The model under review builds one solid part; all positions refer to its coordinate system, in mm. A direction names the side the tool comes from. Round coordinates to 2 decimals unless told otherwise and drop trailing zeros. Order: outer loops, then holes, each group sorted by start corner. A loop starts at its lowest first (then second) coordinate and runs counter-clockwise, first axis right, second up.
Autodesk Inventor part; units mm, degrees
ref_plane "YZ Plane" through (0, 0, 0) normal (1, 0, 0) x (0, 1, 0)
ref_plane "XZ Plane" through (0, 0, 0) normal (0, 1, 0) x (-1, 0, 0)
ref_plane "XY Plane" through (0, 0, 0) normal (0, 0, 1) x (1, 0, 0)
sketch "Skizze1" plane through (0, 0, 0) normal (0, 0, 1) x (1, 0, 0)
  line L0 (2.7, 9.6) -> (2.7, 4)
  arc A0 (2.7, 9.6) -> (2.2, 10.1) centre (2.2, 9.6) ccw
  line L1 (-0.6, 10.1) -> (2.2, 10.1)
  line L2 (-2.3, 10.1) -> (-0.6, 10.1)
  line L3 (-2.3, 10.1) -> (-2.3, 9.1)
  line L4 (-2.3, 9.1) -> (-2.3, 0)
  line L5 (-2.3, 0) -> (-2.3, -1)
  line L6 (-0.6, -1) -> (-2.3, -1)
  line L7 (-0.6, -0.995) -> (0, -0.995)
  line L8 (5.3, -1) -> (-0.6, -1)
  arc A1 (5.3, -1) -> (6.3, 0) centre (5.3, 0) ccw
  line L9 (6.3, 3) -> (6.3, 0)
  arc A2 (6.3, 3) -> (5.3, 4) centre (5.3, 3) ccw
  line L10 (2.7, 4) -> (5.3, 4)
  point P0 (0, 0)
extrude "Extrusion1" add sketch "Skizze1" along normal blind 10.2
sketch "Skizze2" plane through (-2.3, 10.1, 0) normal (0, 1, 0) x (1, 0, 0)
  line L0 (0, -10.2) -> (4.5, -10.2)
  line L1 (0, 0) -> (0, -10.2)
  line L2 (2.3, 0) -> (2.3, -0.9)
  line L3 (2.3, -0.9) -> (1.7, -0.9)
  line L4 (1.7, -0.9) -> (1.7, -1.5)
  line L5 (1.7, -1.5) -> (8.6, -1.5)
  line L6 (8.6, 0) -> (8.6, -10.2)
  line L7 (2.3, -10.2) -> (2.3, -9.3)
  line L8 (2.3, -9.3) -> (1.7, -9.3)
  line L9 (1.7, -9.3) -> (1.7, -8.7)
  line L10 (1.7, -8.7) -> (8.6, -8.7)
  line L11 (8.6, -1.5) -> (8.6, 0)
  line L12 (2.3, 0) -> (8.6, 0)
  line L13 (2.3, -10.2) -> (8.6, -10.2)
  line L14 (8.6, -8.7) -> (8.6, -10.2)
  dimension "d2" = 0.9
  dimension "d3" = 0.6
  dimension "d4" = 0.9
  dimension "d5" = 0.6
  dimension "d6" = 2.3
  dimension "d7" = 2.3
  dimension "d8" = 1.7
  dimension "d9" = 0.6
  dimension "d10" = 1.7
extrude "Extrusion2" cut sketch "Skizze2" against normal blind 12
sketch "Skizze3" plane through (2.7, 4, 8.7) normal (1, 0, 0) x (0, 0, -1)
  line L0 (0, 5.6) -> (0, 0)
  line L1 (7.2, 0) -> (0, 0)
  line L2 (7.2, 0) -> (7.2, 5.6)
  line L3 (7.2, 5.6) -> (0, 5.6)
  line L4 (7.2, 6.1) -> (0, 6.1)
  line L5 (-1.5, -5) -> (-1.5, 6.1)
  point P0 (8.7, -4)
  point P1 (3.55, 2.55)
  dimension "d13" = 3.55
  dimension "d14" = 5.05
sketch "Skizze4" plane through (-2.3, -1, 0) normal (-1, 0, 0) x (0, 0, 1)
  line L0 (10.2, 0) -> (10.2, 11.1)
  line L1 (0, 11.1) -> (10.2, 11.1)
  line L2 (0, 0) -> (0, 11.1)
  line L3 (10.2, 11.1) -> (10.2, 0)
  line L4 (10.2, 0) -> (0, 0)
  line L5 (0, 0) -> (0, 11.1)
  line L6 (0, 11.1) -> (10.2, 11.1)
  line L7 (10.2, 11.1) -> (10.2, 0)
  line L8 (10.2, 0) -> (0, 0)
  line L9 (0, 0) -> (0, 11.1)
  line L10 (0, 11.1) -> (10.2, 11.1)
  line L11 (10.2, 0) -> (10.2, 11.1)
  line L12 (0, 11.1) -> (10.2, 11.1)
  line L13 (0, 0) -> (0, 11.1)
  line L14 (0, 0) -> (10.2, 0)
  line L15 (8.7, 10.6) -> (8.7, 5)
  line L16 (1.5, 5) -> (8.7, 5)
  line L17 (1.5, 5) -> (1.5, 10.6)
  line L18 (1.5, 10.6) -> (8.7, 10.6)
  point P0 (0, 1)
  point P1 (5.1, 7.55)
  dimension "d15" = 3.55
  dimension "d16" = 5.1
  dimension "d17" = 5.1
hole "Hole1" at (-2.3, 6.55, 5.1) direction (1, 0, 0) diameter 2.013 end through all countersink diameter 4 countersink angle 90
sketch "Skizze5" plane through (2.2, 10.1, 1.5) normal (0, 0, -1) x (-1, 0, 0)
  line L0 (-4.1, -10.1) -> (-4.1, -7.1)
  line L1 (2.8, -11.1) -> (-3.1, -11.1)
  line L2 (-3.1, -6.1) -> (-0.5, -6.1)
  line L3 (2.2, 0) -> (2.2, -11.1)
  point P0 (2.2, -10.1)
  point P1 (-1.6, -8.6)
  dimension "d25" = 2.5
  dimension "d26" = 2.5
  dimension "d27" = 2.5
  dimension "d28" = 3.8
sketch "Skizze6" plane through (-0.6, 10.1, 8.7) normal (0, 0, 1) x (1, 0, 0)
  line L0 (6.9, -7.1) -> (6.9, -10.1)
  line L1 (3.3, -6.1) -> (5.9, -6.1)
  line L2 (0.6, -11.1) -> (0.6, 0)
  point P0 (0.6, -10.1)
  point P1 (4.4, -8.6)
  dimension "d29" = 2.5
  dimension "d30" = 2.5
  dimension "d31" = 3.8
hole "Hole2" at (3.8, 1.5, 8.7) direction (0, 0, -1) diameter 2.013 depth 6 tip angle 118 countersink diameter 4 countersink angle 90
hole "Hole3" at (3.8, 1.5, 1.5) direction (0, 0, 1) diameter 2.013 depth 6 tip angle 118 countersink diameter 4 countersink angle 90
sketch "Skizze7" plane through (-2.3, 10.1, 10.2) normal (0, 1, 0) x (1, 0, 0)
  line L0 (0, 10.2) -> (2.3, 10.2)
  line L1 (0, 10.2) -> (0, 0)
  line L2 (0, 0) -> (2.3, 0)
  line L3 (0, 7.65) -> (0.2, 7.65)
  line L4 (0.2, 7.65) -> (0.2, 2.55)
  line L5 (0.2, 2.55) -> (0, 2.55)
  line L6 (0, 7.65) -> (0, 2.55)
  dimension "d46" = 2.55
  dimension "d47" = 2.55
  dimension "d48" = 0.2
extrude "Extrusion3" cut sketch "Skizze7" against normal blind 12
fillet "Rundung1" radius 0.5 1 edges at (-1.15, 10.1, 10.2)
fillet "Rundung2" radius 0.5 3 edges at (-1.15, 10.1, 0) (-1.15, -1, 0) (-1.15, -1, 10.2)
properties part number "4. Leiterplattenhalter_Links"
(1) We need section D-D (z = 8). Give the boundary of the cut face in (x, y), and give its area (3 significant figures).
(2) We need section A-A (y = 1.5). Give the boundary of the cut face in (x, z), and give its area (3 significant figures).
(3) To check wall thickness, follow L1, parallel to Y at x = 3.8, z = 7.6; L2, parallel to Z at x = -0.5, y = 7; L3, parallel to Y at x = -0.3, z = 5.1. State the ranges of each line that lie inside material, in increasing order.
(4) Clearance check with flat-ended pins moving along their axes: P1, Ø3.5, axis at x = 3, y = 2.5, coming from the -Z side; P2, Ø0.7, axis at y = 3.5, z = 1, coming from the +X side; P3, Ø1.5, axis at y = 2, z = 4.5, coming from the -X side. State where each tip first meets the part, or that it passes through.
(5) We need section C-C (x = 1.25). Give the boundary of the cut face in (y, z), and give its area (3 significant figures).
(6) We need section B-B (z = 5.1). Give the boundary of the cut face in (x, y), and give its area (3 significant figures).
(7) The part is to be moulded in two halves that separate along Z. For faces 1 (the flat face through (0, 10.1, 5)), 2 (the cylindrical face through (1, 7, 6)), 3 (the flat face through (-1, 5, 10.2)), 4 (the flat face through (1, 5, 1.5)), say which applies: pulls with the +Z half, pulls with the -Z half, needs draft (parallel to the pull), parting line crosses it, or undercut.
(8) Tool access review of faces 5 (the flat face through (0, 5, 10)), 6 (the flat face through (-2.1, 4.6, 5.1)), 7 (the flat face through (6.3, 2, 5)), 8 (the flat face through (4, 4, 5)), 9 (the flat face through (0, 4.6, 0.4)): name each direction out of +Z, -Z, +X, -X, +Y, -Y from which nothing blocks a thin tool from reaching the whole face with its end or side.
Verdict:
1. outline: (-2.3, -1) - (5.3, -1) arc R1 ccw to (6.3, 0) - (6.3, 3) arc R1 ccw to (5.3, 4) - (2.7, 4) - (2.7, 9.6) arc R0.5 ccw to (2.2, 10.1) - (-2.3, 10.1) - close; hole circle Ø2.6 at (3.8, 1.5)
1. area: 67.7 mm2
2. outline: (-2.3, 0) - (0, 0) - (0, 0.9) - (-0.6, 0.9) - (-0.6, 1.5) - (1.8, 1.5) - (2.79, 2.49) - (2.79, 7.71) - (1.8, 8.7) - (-0.6, 8.7) - (-0.6, 9.3) - (0, 9.3) - (0, 10.2) - (-2.3, 10.2) - (-2.3, 7.65) - (-2.1, 7.65) - (-2.1, 2.55) - (-2.3, 2.55) - close; (4.81, 2.49) - (5.8, 1.5) - (6.3, 1.5) - (6.3, 8.7) - (5.8, 8.7) - (4.81, 7.71) - close
2. area: 50.6 mm2
3. L1: y = -1 to 0.49, 2.51 to 4
3. L2: z = 0 to 0.9, 1.5 to 4.2, 6 to 8.7, 9.3 to 10.2
3. L3: y = -1 to 5.54, 7.56 to 10.1
4. P1: stops at z = 1.5
4. P2: stops at x = 0
4. P3: stops at x = -2.1
5. outline: (-1, 1.5) - (10.1, 1.5) - (10.1, 8.7) - (-1, 8.7) - close; hole circle Ø2.01 at (6.55, 5.1)
5. area: 76.7 mm2
6. outline: (-2.1, -1) - (5.3, -1) arc R1 ccw to (6.3, 0) - (6.3, 3) arc R1 ccw to (5.3, 4) - (2.7, 4) - (2.7, 5.54) - (-1.31, 5.54) - (-2.1, 4.75) - close; (-2.1, 8.35) - (-1.31, 7.56) - (2.7, 7.56) - (2.7, 9.6) arc R0.5 ccw to (2.2, 10.1) - (-2.1, 10.1) - close; hole circle Ø2.01 at (3.8, 1.5)
6. area: 57.3 mm2
7. face 1: needs draft
7. face 2: undercut
7. face 3: pulls with the +Z half
7. face 4: undercut
8. face 5: +Z, +X, +Y, -Y
8. face 6: -X, +Y, -Y
8. face 7: +Z, -Z, +X, +Y, -Y
8. face 8: +Z, -Z, +X, +Y
8. face 9: -Z, +X, +Y, -Y
